Source: CAD feature listing. Evaluate the final solid. Frame: model axes, mm. Face numbers are marked on the shaded views. A direction names the side the tool comes from. Round coordinates to 2 decimals unless told otherwise and drop trailing zeros. Order: outer loops, then holes, each group sorted by start corner. A loop starts at its lowest first (then second) coordinate and runs counter-clockwise, first axis right, second up. Notation, with made-up numbers: (89.5, 44) -> (125.5, 44) arc R11 cw to (125.5, 50) -> close; hole circle Ø4 at (19.25, 55). An arc over 180 degrees is marked (long way). Write item = value, one per line. Start each with the question number.
(1) Reachability of the marked faces 1, 2 and 3 from +Z, -Z, +X, -X, +Y, -Y: full face, straight path, thin tool, end or side. Return the list, or none.
(2) Cut plane A-A on z = 24. Return the cut outline in (x, y), then the cut area to 3 significant figures.
(3) Cut plane D-D on y = -10.5. Return the cut outline in (x, z).
(4) Cut plane B-B on x = 0. Return the cut outline in (y, z).
(5) Contact query for flat-ended pins moving along their axis: pin 1 Ø14.5 at (x, y) = (1.5, 12) entering from -Z; pin 2 Ø21 at (y, z) = (10, -26.5) entering from +X; pin 3 Ø5.5 at (x, z) = (-1.5, 22) entering from -Y; pin 4 Ø5 at (x, z) = (-28.5, -11) entering from -Y. Output: stop coordinate, or through.
(6) Draft query along Z for the marked faces 4, 5, 6 and 7. Return one class per face: released by +Z, released by -Z, zero draft, split by the parting line, or undercut.
(7) Ray query, line 1 (X direction, y = 1.95, z = 24); line 2 (Z direction, x = 5, y = 3); line 3 (X direction, y = 17.5, z = 10). Return the intervals inside material, ascending.
from build123d import *

# Parameters (mm, degrees)
BOSS_EXTRUDE1_DEPTH = 20
BOSS_EXTRUDE2_DEPTH = 2
SKETCH5_W           = 20
SKETCH5_H           = 20
SKETCH5_R           = 3.5
BOSS_EXTRUDE3_DEPTH = 22
SKETCH6_W           = 18
SKETCH6_H           = 19
CUT_EXTRUDE1_DEPTH  = 20
SKETCH7_W           = 20
SKETCH7_H           = 19
CUT_EXTRUDE2_DEPTH  = 1.5
FILLET1_R           = 3
SKETCH8_R           = 15.7
CUT_EXTRUDE3_DEPTH  = 121.5
BOSS_EXTRUDE6_START = 13.4
BOSS_EXTRUDE6_DEPTH = 13.4
SKETCH12_W          = 1
SKETCH12_H          = 30.481485494
BOSS_EXTRUDE7_DEPTH = 23.4
CUT_EXTRUDE4_DEPTH  = 93.4


with BuildPart() as part:
    # Sketch3 → Boss-Extrude1 (new body)
    with BuildSketch(Plane(origin=(0, 0, 0), x_dir=(1, 0, 0), z_dir=(0, 1, 0))):
        with BuildLine():
            Line((36, -26), (36, 26))
            ThreePointArc((36, 26), (33.071067812, 33.071067812), (26, 36))
            Line((26, 36), (-26, 36))
            ThreePointArc((-26, 36), (-33.071067812, 33.071067812), (-36, 26))
            Line((-36, 26), (-36, -26))
            ThreePointArc((-36, -26), (-33.071067812, -33.071067812), (-26, -36))
            Line((-26, -36), (26, -36))
            ThreePointArc((26, -36), (33.071067812, -33.071067812), (36, -26))
        make_face()
        with BuildLine():
            Line((-35, 25), (-35, -25))
            ThreePointArc((-35, -25), (-32.071067812, -32.071067812), (-25, -35))
            Line((-25, -35), (25, -35))
            ThreePointArc((25, -35), (32.071067812, -32.071067812), (35, -25))
            Line((35, -25), (35, 25))
            ThreePointArc((35, 25), (32.071067812, 32.071067812), (25, 35))
            Line((25, 35), (-25, 35))
            ThreePointArc((-25, 35), (-32.071067812, 32.071067812), (-35, 25))
        make_face(mode=Mode.SUBTRACT)
    extrude(amount=BOSS_EXTRUDE1_DEPTH)

    # Sketch4 → Boss-Extrude2 (add)
    with BuildSketch(Plane(origin=(0, 20, 0), x_dir=(1, 0, 0), z_dir=(0, 1, 0))):
        with BuildLine():
            Line((0, 36), (0, 0))
            Line((0, 0), (-36, 0))
            Line((-36, 0), (-36, -26))
            ThreePointArc((-36, -26), (-33.071067812, -33.071067812), (-26, -36))
            Line((-26, -36), (26, -36))
            ThreePointArc((26, -36), (33.071067812, -33.071067812), (36, -26))
            Line((36, -26), (36, 26))
            ThreePointArc((36, 26), (33.071067812, 33.071067812), (26, 36))
            Line((26, 36), (0, 36))
        make_face()
        with BuildLine():
            Line((-36, 0), (0, 0))
            Line((0, 0), (0, 36))
            Line((0, 36), (-26, 36))
            ThreePointArc((-26, 36), (-33.071067812, 33.071067812), (-36, 26))
            Line((-36, 26), (-36, 0))
        make_face()
    extrude(amount=BOSS_EXTRUDE2_DEPTH)

    # Sketch5 → Boss-Extrude3 (add)
    # profile 1 of 2: a face of its own
    with BuildSketch(Plane(origin=(0, 22, 0), x_dir=(1, 0, 0), z_dir=(0, 1, 0))):
        with Locations((0, 26)):
            Rectangle(SKETCH5_W, SKETCH5_H)
        with Locations(Location((0, 24, 0), (0, 0, 270))):
            Circle(SKETCH5_R, mode=Mode.SUBTRACT)
    # profile 2 of 2: a face of its own
    with BuildSketch(Plane(origin=(0, 22, 0), x_dir=(1, 0, 0), z_dir=(0, 1, 0))):
        with Locations((0, -26)):
            Rectangle(SKETCH5_W, SKETCH5_H)
        with Locations(Location((0, -24, 0), (0, 0, 270))):
            Circle(SKETCH5_R, mode=Mode.SUBTRACT)
    extrude(amount=-BOSS_EXTRUDE3_DEPTH)

    # Sketch6 → Cut-Extrude1 (cut)
    with BuildSketch(Plane(origin=(0, 22, 0), x_dir=(1, 0, 0), z_dir=(0, 1, 0))):
        Polygon((0, -17), (-9, -17), (-9, -36), (9, -36), (9, -17), align=None)
        with Locations((0, 26.5)):
            Rectangle(SKETCH6_W, SKETCH6_H)
    extrude(amount=-CUT_EXTRUDE1_DEPTH, mode=Mode.SUBTRACT)

    # Sketch7 → Cut-Extrude2 (cut)
    with BuildSketch(Plane(origin=(0, 0, 0), x_dir=(-1, 0, 0), z_dir=(0, -1, 0))):
        with Locations((0, 25.5)):
            Rectangle(SKETCH7_W, SKETCH7_H)
        with Locations((0, -25.5)):
            Rectangle(SKETCH7_W, SKETCH7_H)
    extrude(amount=-CUT_EXTRUDE2_DEPTH, mode=Mode.SUBTRACT)

    # Fillet1
    fillet1_edges = [part.edges().sort_by_distance(p)[0] for p in [
        (-17.5, 22, 36),
        (-17.5, 22, -36),
        (-33.071067812, 22, 33.071067812),
        (17.5, 22, 36),
        (36, 22, 0),
        (33.071067812, 22, -33.071067812),
        (17.5, 22, -36),
        (-33.071067812, 22, -33.071067812),
        (-36, 22, 0),
        (33.071067812, 22, 33.071067812),
    ]]
    fillet(fillet1_edges, radius=FILLET1_R)

    # Sketch8 → Cut-Extrude3 (cut)
    with BuildSketch(Plane(origin=(36, 0, 0), x_dir=(0, 0, -1), z_dir=(1, 0, 0))):
        with Locations((0, -12.6)):
            Circle(SKETCH8_R)
    extrude(amount=-CUT_EXTRUDE3_DEPTH, mode=Mode.SUBTRACT)

    # Sketch9 → Boss-Extrude6 (add)
    with BuildSketch(Plane(origin=(0, 0, 0), x_dir=(-1, 0, 0), z_dir=(0, -1, 0)).offset(BOSS_EXTRUDE6_START)):
        with BuildLine():
            Line((26, 36), (-26, 36))
            ThreePointArc((-26, 36), (-33.071067812, 33.071067812), (-36, 26))
            Line((-36, 26), (-36, -26))
            ThreePointArc((-36, -26), (-33.071067812, -33.071067812), (-26, -36))
            Line((-26, -36), (26, -36))
            ThreePointArc((26, -36), (33.071067812, -33.071067812), (36, -26))
            Line((36, -26), (36, 26))
            ThreePointArc((36, 26), (33.071067812, 33.071067812), (26, 36))
        make_face()
        with BuildLine():
            ThreePointArc((25, 35), (32.071067812, 32.071067812), (35, 25))
            Line((35, 25), (35, -25))
            ThreePointArc((35, -25), (32.071067812, -32.071067812), (25, -35))
            Line((25, -35), (-25, -35))
            ThreePointArc((-25, -35), (-32.071067812, -32.071067812), (-35, -25))
            Line((-35, -25), (-35, 25))
            ThreePointArc((-35, 25), (-32.071067812, 32.071067812), (-25, 35))
            Line((-25, 35), (25, 35))
        make_face(mode=Mode.SUBTRACT)
    extrude(amount=-BOSS_EXTRUDE6_DEPTH)

    # Sketch12 → Boss-Extrude7 (add)
    with BuildSketch(Plane.XZ.offset(13.4)):
        with Locations((-35.5, 0.993188546)):
            Rectangle(SKETCH12_W, SKETCH12_H)
        with Locations((35.5, 0.993188546)):
            Rectangle(SKETCH12_W, SKETCH12_H)
    extrude(amount=-BOSS_EXTRUDE7_DEPTH)

    # Sketch13 → Cut-Extrude4 (cut)
    with BuildSketch(Plane.ZY.offset(36)):
        with BuildLine():
            Line((-10.476256632, -13.4), (0, -13.4))
            Line((0, -13.4), (0, -9.460687563))
            ThreePointArc((0, -9.460687563), (-5.596207097, -10.478064604), (-10.476256632, -13.4))
        make_face()
        with BuildLine():
            Line((0, -9.460687563), (0, -13.4))
            Line((0, -13.4), (10.476256632, -13.4))
            ThreePointArc((10.476256632, -13.4), (5.596207097, -10.478064604), (0, -9.460687563))
        make_face()
    extrude(amount=-CUT_EXTRUDE4_DEPTH, mode=Mode.SUBTRACT)


solid = part.part
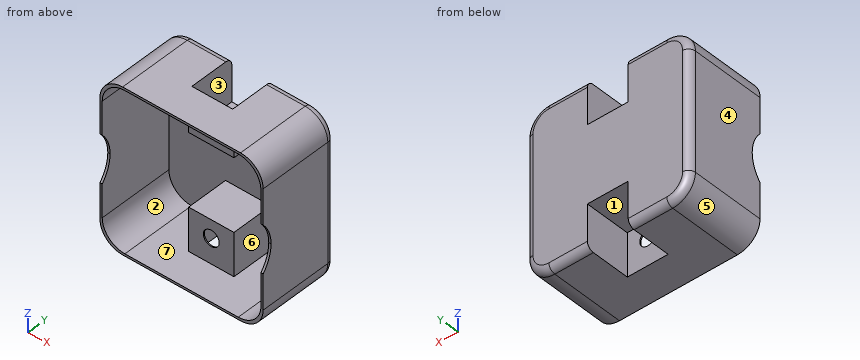
Evaluation:
q1.face_1 = -Z, +Y
q1.face_2 = -Y
q1.face_3 = +Z, +Y
q2.outline = (-36, -13.4) -> (-35, -13.4) -> (-35, 20) -> (-10, 20) -> (-10, 1.5) -> (-3.5, 1.5) -> (-3.5, 2) -> (-9, 2) -> (-9, 22) -> (-33, 22) arc R3 ccw to (-36, 19) -> close; (3.5, 1.5) -> (10, 1.5) -> (10, 20) -> (35, 20) -> (35, -13.4) -> (36, -13.4) -> (36, 19) arc R3 ccw to (33, 22) -> (9, 22) -> (9, 2) -> (3.5, 2) -> close
q2.area = 213 mm^2
q3.outline = (-36, -26) arc R10 ccw to (-26, -36) -> (26, -36) arc R10 ccw to (36, -26) -> (36, -5.65) -> (35, -5.65) -> (35, -25) arc R10 cw to (25, -35) -> (-25, -35) arc R10 cw to (-35, -25) -> (-35, -5.65) -> (-36, -5.65) -> close; (-36, 5.65) -> (-35, 5.65) -> (-35, 25) arc R10 cw to (-25, 35) -> (25, 35) arc R10 cw to (35, 25) -> (35, 5.65) -> (36, 5.65) -> (36, 26) arc R10 ccw to (26, 36) -> (-26, 36) arc R10 ccw to (-36, 26) -> close
q4.outline = (-13.4, -36) -> (2, -36) -> (2, -27.5) -> (1.5, -27.5) -> (1.5, -35) -> (-13.4, -35) -> close; (-13.4, 35) -> (1.5, 35) -> (1.5, 27.5) -> (2, 27.5) -> (2, 36) -> (-13.4, 36) -> close; (1.5, -20.5) -> (2, -20.5) -> (2, -17) -> (22, -17) -> (22, 17) -> (2, 17) -> (2, 20.5) -> (1.5, 20.5) -> (1.5, 16) -> (20, 16) -> (20, -16) -> (1.5, -16) -> close
q5.pin_1 = -17
q5.pin_2 = 36
q5.pin_3 = 1.5
q5.pin_4 = 20
q6.face_4 = zero draft
q6.face_5 = released by -Z
q6.face_6 = undercut
q6.face_7 = undercut
q7.line_1 = -36 to -35, -10 to -3.5, 3.5 to 10, 35 to 36
q7.line_2 = -17 to -16, 16 to 17
q7.line_3 = -36 to -35, 35 to 36
